Here's how the part is built. I have some questions about the finished solid (model axes, mm). Face numbers are marked on the shaded views. Give positions to 0.01 mm unless a question says otherwise; leave off trailing zeros. Loops run counter-clockwise (first coordinate to the right, second up) from the corner with the lowest first, then second, coordinate; pieces in that order, holes last. Notation, with made-up numbers: M -13.5,20.5 L 15.5,20.5 A23 ccw 15.5,36.5 Z; hole C 34,53.25 d3. An arc over 180 degrees is marked long. Answer as CSV lines item,"result". Start each with the question number.
Item 1: I want a section at A-A on x = 0. List the corners of the cut face in (y, z) for me, plus the area to 3 significant figures.
Item 2: If we mould it in two halves opening along X, with no side actions, what happens to the marked faces 1, 2 and 3? For each: released by +X, released by -X, zero draft, split by the parting line, or undercut.
Item 3: If I drill on line 1 along Z through (x, y) = (0, -8.25); line 2 along Y through (x, z) = (46, -33.5); line 3 along X through (y, z) = (-20.25, 7), over which ranges is the centre line in solid material (lowest first)? Write a range as from..to.
Item 4: I want a section at C-C on z = -22. List the corners of the cut face in (x, y) for me, plus the area to 3 significant figures.
Item 5: I want a section at B-B on y = -9.75. List the corners of the cut face in (x, z) for me, plus the area to 3 significant figures.
from build123d import *

# Parameters (mm, degrees)
F0_W     = 105.252586
F0_H     = 76.403916
F1_DEPTH = 30
F2_R     = 5
F4_D     = 50


with BuildPart() as f1:
    # F0 (on Front) → F1 (new body)
    with BuildSketch(Plane.XZ):
        Rectangle(F0_W, F0_H)
    extrude(amount=F1_DEPTH)

    # F2
    f2_edges = [f1.edges().sort_by_distance(p)[0] for p in [
        (0, -30, 38.201958),
        (-52.626293, -30, 0),
        (0, -30, -38.201958),
        (52.626293, -30, 0),
        (-52.626293, -15, 38.201958),
        (-52.626293, -15, -38.201958),
        (52.626293, -15, 38.201958),
        (52.626293, -15, -38.201958),
    ]]
    fillet(f2_edges, radius=F2_R)

    # F4 (through all)
    with Locations(Plane.XZ.offset(30)):
        with Locations((0, 0)):
            Hole(F4_D / 2)


solid = f1.part
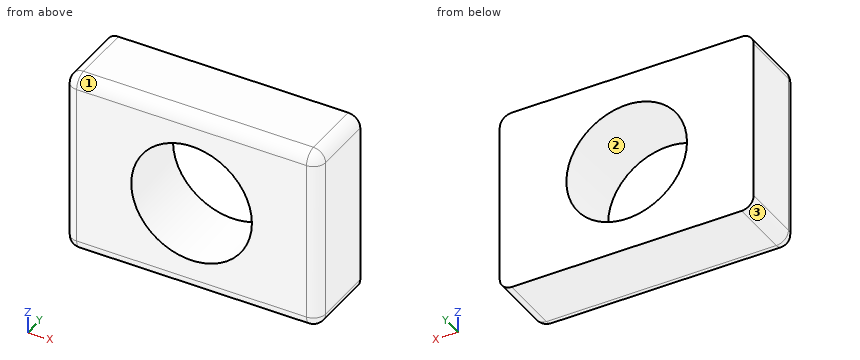
Result:
1,outline,"M -30,-33.2 A5 ccw -25,-38.2 L 0,-38.2 L 0,-25 L -30,-25 Z; M -30,25 L 0,25 L 0,38.2 L -25,38.2 A5 ccw -30,33.2 Z"
1,area,"781 mm^2"
2,face 1,"zero draft"
2,face 2,"undercut"
2,face 3,"released by -X"
3,line 1,"-38.2..-25, 25..38.2"
3,line 2,"-29.99..0"
3,line 3,"-52.63..-24, 24..52.63"
4,outline,"M -52.63,-25 A5 ccw -47.63,-30 L -11.87,-30 L -11.87,0 L -52.63,0 Z; M 11.87,-30 L 47.63,-30 A5 ccw 52.63,-25 L 52.63,0 L 11.87,0 Z"
4,area,"2,430 mm^2"
5,outline,"M -52.63,-33.2 A5 ccw -47.63,-38.2 L 47.63,-38.2 A5 ccw 52.63,-33.2 L 52.63,33.2 A5 ccw 47.63,38.2 L -47.63,38.2 A5 ccw -52.63,33.2 Z; hole C 0,0 d50"
5,area,"6,060 mm^2"
